```python
from build123d import *

# Parameters (mm, degrees)
ESQUISSE1_W              = 85
ESQUISSE1_H              = 73
BOSS_EXTRU_2_DEPTH       = 1
ESQUISSE6_W              = 35
ESQUISSE6_H              = 73
BOSS_EXTRU_4_DEPTH       = 1
ESQUISSE8_W              = 35
ESQUISSE8_H              = 73
BOSS_EXTRU_6_DEPTH       = 1
ESQUISSE10_W             = 12
ESQUISSE10_H             = 11
ENL_V_MAT_EXTRU_1_DEPTH  = 1
ESQUISSE11_W             = 15
ESQUISSE11_H             = 13
ENL_V_MAT_EXTRU_2_DEPTH  = 1
ESQUISSE13_W             = 87
ESQUISSE13_H             = 35
BOSS_EXTRU_8_DEPTH       = 1
ESQUISSE14_W             = 12
ESQUISSE14_H             = 16
ENL_V_MAT_EXTRU_3_DEPTH  = 1
ESQUISSE18_W             = 12
ESQUISSE18_H             = 16
ENL_V_MAT_EXTRU_5_DEPTH  = 1
ESQUISSE20_W             = 12
ESQUISSE20_H             = 16
ENL_V_MAT_EXTRU_6_DEPTH  = 1
ESQUISSE21_W             = 12
ESQUISSE21_H             = 16
ENL_V_MAT_EXTRU_7_DEPTH  = 1
ESQUISSE22_R             = 3.5
ENL_V_MAT_EXTRU_8_DEPTH  = 1
ESQUISSE24_R             = 3.5
ENL_V_MAT_EXTRU_10_DEPTH = 1
ESQUISSE25_W             = 87
ESQUISSE25_H             = 35
BOSS_EXTRU_11_DEPTH      = 1
ESQUISSE23_R             = 3.5
ENL_V_MAT_EXTRU_12_DEPTH = 1
ESQUISSE26_W             = 77
ESQUISSE26_H             = 21
ENL_V_MAT_EXTRU_13_DEPTH = 1


with BuildPart() as part:
    # Esquisse1 → Boss.-Extru.2 (new body)
    with BuildSketch(Plane.XY):
        with Locations((-89.704998798, 36.5)):
            Rectangle(ESQUISSE1_W, ESQUISSE1_H)
    extrude(amount=BOSS_EXTRU_2_DEPTH)

    # Esquisse6 → Boss.-Extru.4 (add)
    with BuildSketch(Plane(origin=(-47.204998798, 0, 0), x_dir=(0, 0, -1), z_dir=(1, 0, 0))):
        with Locations((-17.5, 36.5)):
            Rectangle(ESQUISSE6_W, ESQUISSE6_H)
    extrude(amount=BOSS_EXTRU_4_DEPTH)

    # Esquisse8 → Boss.-Extru.6 (add)
    with BuildSketch(Plane.ZY.offset(132.204998798)):
        with Locations((17.5, 36.5)):
            Rectangle(ESQUISSE8_W, ESQUISSE8_H)
    extrude(amount=BOSS_EXTRU_6_DEPTH)

    # Esquisse10 → Enlèv. mat.-Extru.1 (cut)
    with BuildSketch(Plane.ZY.offset(133.204998798)):
        with Locations((8, 59.5)):
            Rectangle(ESQUISSE10_W, ESQUISSE10_H)
    extrude(amount=-ENL_V_MAT_EXTRU_1_DEPTH, mode=Mode.SUBTRACT)

    # Esquisse11 → Enlèv. mat.-Extru.2 (cut)
    with BuildSketch(Plane.ZY.offset(133.204998798)):
        with Locations((9.5, 30.5)):
            Rectangle(ESQUISSE11_W, ESQUISSE11_H)
    extrude(amount=-ENL_V_MAT_EXTRU_2_DEPTH, mode=Mode.SUBTRACT)

    # Esquisse13 → Boss.-Extru.8 (add)
    with BuildSketch(Plane(origin=(0, 73, 0), x_dir=(1, 0, 0), z_dir=(0, 1, 0))):
        with Locations((-89.704998798, -17.5)):
            Rectangle(ESQUISSE13_W, ESQUISSE13_H)
    extrude(amount=BOSS_EXTRU_8_DEPTH)

    # Esquisse14 → Enlèv. mat.-Extru.3 (cut)
    with BuildSketch(Plane(origin=(0, 74, 0), x_dir=(1, 0, 0), z_dir=(0, 1, 0))):
        with Locations((-122.207040337, -26)):
            Rectangle(ESQUISSE14_W, ESQUISSE14_H)
    extrude(amount=-ENL_V_MAT_EXTRU_3_DEPTH, mode=Mode.SUBTRACT)

    # Esquisse18 → Enlèv. mat.-Extru.5 (cut)
    with BuildSketch(Plane(origin=(0, 74, 0), x_dir=(1, 0, 0), z_dir=(0, 1, 0))):
        with Locations((-108.207040337, -26)):
            Rectangle(ESQUISSE18_W, ESQUISSE18_H)
    extrude(amount=-ENL_V_MAT_EXTRU_5_DEPTH, mode=Mode.SUBTRACT)

    # Esquisse20 → Enlèv. mat.-Extru.6 (cut)
    with BuildSketch(Plane(origin=(0, 74, 0), x_dir=(1, 0, 0), z_dir=(0, 1, 0))):
        with Locations((-94.207040337, -26)):
            Rectangle(ESQUISSE20_W, ESQUISSE20_H)
    extrude(amount=-ENL_V_MAT_EXTRU_6_DEPTH, mode=Mode.SUBTRACT)

    # Esquisse21 → Enlèv. mat.-Extru.7 (cut)
    with BuildSketch(Plane(origin=(0, 74, 0), x_dir=(1, 0, 0), z_dir=(0, 1, 0))):
        with Locations((-80.207040337, -26)):
            Rectangle(ESQUISSE21_W, ESQUISSE21_H)
    extrude(amount=-ENL_V_MAT_EXTRU_7_DEPTH, mode=Mode.SUBTRACT)

    # Esquisse22 → Enlèv. mat.-Extru.8 (cut)
    with BuildSketch(Plane.XY.offset(1)):
        with Locations((-128.334603856, 69.17039525)):
            Circle(ESQUISSE22_R)
    extrude(amount=-ENL_V_MAT_EXTRU_8_DEPTH, mode=Mode.SUBTRACT)

    # Esquisse24 → Enlèv. mat.-Extru.10 (cut)
    with BuildSketch(Plane.XY.offset(1)):
        with Locations((-69.71638406, 68.525894508)):
            Circle(ESQUISSE24_R)
    extrude(amount=-ENL_V_MAT_EXTRU_10_DEPTH, mode=Mode.SUBTRACT)

    # Esquisse25 → Boss.-Extru.11 (add)
    with BuildSketch(Plane.XZ):
        with Locations((-89.704998798, 17.5)):
            Rectangle(ESQUISSE25_W, ESQUISSE25_H)
    extrude(amount=BOSS_EXTRU_11_DEPTH)

    # Esquisse23 → Enlèv. mat.-Extru.12 (cut)
    with BuildSketch(Plane.XY.offset(1)):
        with Locations((-128.228777758, 19.66052326)):
            Circle(ESQUISSE23_R)
    extrude(amount=-ENL_V_MAT_EXTRU_12_DEPTH, mode=Mode.SUBTRACT)

    # Esquisse26 → Enlèv. mat.-Extru.13 (cut)
    with BuildSketch(Plane.XZ.offset(1)):
        with Locations((-84.785991567, 10.567106243)):
            Rectangle(ESQUISSE26_W, ESQUISSE26_H)
    extrude(amount=-ENL_V_MAT_EXTRU_13_DEPTH, mode=Mode.SUBTRACT)


solid = part.part
```
Model file for the job. Use its own axes, mm. A direction names the side the tool comes from. Round coordinates to 2 decimals unless told otherwise and drop trailing zeros. Write each loop counter-clockwise with the first axis right and the second up, starting at its lowest first coordinate (ties: lowest second). Pieces come first, ordered by that corner, then holes. Notation, with made-up numbers: (4, 44) - (39, 44) arc R21 cw to (39, 82) - close; hole circle Ø9 at (-18.5, 9). An arc over 180 degrees is marked (long way). Use CSV: the item, a comma, the result in double quotes. Start each with the question number.
Item 1: Band-saw the part on D-D (z = 28). Write the cut outline in (x, y) (3 decimals), and give its area (3 significant figures).
Item 2: Pin check, flat tips, straight feed: P1, Ø1.1, axis at x = -133, y = 28, coming from the -Z side; P2, Ø1, axis at x = -123.5, z = 20.5, coming from the +Y side. Stop position of each tip, or through.
Item 3: Tool access for faces 4 (the face through (-90, 37, 0)), 5 (the face through (-81, 73, 14)): list every direction of +Z, -Z, +X, -X, +Y, -Y with a clear straight run to the whole face (end or side of a thin tool).
Item 4: Two-plate mould, pull along Y, no slides. Class faces 1 (the face through (-131.83, 69.32, 0.51)), 2 (the face through (-85, 0, 0.5)), 3 (the face through (-90, 74, 13)): released by +Y, released by -Y, zero draft, split by the parting line, or undercut.
Item 5: Drill centre lines: L1, parallel to Y at x = -86.5, z = 29.5; L2, parallel to X at y = 59.5, z = 33 (3 decimals); L3, parallel to Y at x = -65, z = 13. Where is each one in solid material? Low to high. Write a range as [from, to].
Item 6: Band-saw the part on C-C (x = -92.5). Write the cut outline in (y, z), and give its area (3 significant figures).
Item 7: Band-saw the part on B-B (y = 64). Write the cut outline in (x, z) (3 decimals).
Item 8: Band-saw the part on A-A (z = 13). Write the cut outline in (x, y) (3 decimals), and give its area (3 significant figures).
Checked values:
1,outline,"(-133.205, -1) - (-46.205, -1) - (-46.205, 74) - (-74.207, 74) - (-74.207, 73) - (-47.205, 73) - (-47.205, 0) - (-132.205, 0) - (-132.205, 73) - (-128.207, 73) - (-128.207, 74) - (-133.205, 74) - close; (-116.207, 73) - (-114.207, 73) - (-114.207, 74) - (-116.207, 74) - close; (-102.207, 73) - (-100.207, 73) - (-100.207, 74) - (-102.207, 74) - close; (-88.207, 73) - (-86.207, 73) - (-86.207, 74) - (-88.207, 74) - close"
1,area,"272 mm²"
2,P1,"stops at z = 0"
2,P2,"stops at y = 0"
3,face 4,"-Z, +X, -X, +Y, -Y"
3,face 5,"+Z"
4,face 1,"undercut"
4,face 2,"released by -Y"
4,face 3,"released by +Y"
5,L1,"y = [-1, 0], [73, 74]"
5,L2,"x = [-133.205, -132.205], [-47.205, -46.205]"
5,L3,"y = [73, 74]"
6,outline,"(-1, 0) - (74, 0) - (74, 18) - (73, 18) - (73, 1) - (0, 1) - (0, 0.07) - (-1, 0.07) - close; (-1, 21.07) - (0, 21.07) - (0, 35) - (-1, 35) - close; (73, 34) - (74, 34) - (74, 35) - (73, 35) - close"
6,area,"106 mm²"
7,outline,"(-133.205, 0) - (-46.205, 0) - (-46.205, 35) - (-47.205, 35) - (-47.205, 1) - (-132.205, 1) - (-132.205, 2) - (-133.205, 2) - close; (-133.205, 14) - (-132.205, 14) - (-132.205, 35) - (-133.205, 35) - close"
8,outline,"(-133.205, -1) - (-123.286, -1) - (-123.286, 0) - (-132.205, 0) - (-132.205, 24) - (-133.205, 24) - close; (-133.205, 37) - (-132.205, 37) - (-132.205, 54) - (-133.205, 54) - close; (-133.205, 65) - (-132.205, 65) - (-132.205, 73) - (-47.205, 73) - (-47.205, 0) - (-46.286, 0) - (-46.286, -1) - (-46.205, -1) - (-46.205, 74) - (-133.205, 74) - close"
8,area,"219 mm²"
